```python
from build123d import *

# Parameters (mm, degrees)
SKETCH_R          = 2
PAD_DEPTH         = 8
SKETCH001_R       = 3.05
POCKET_DEPTH      = 0.001
POCKET_DEPTH_BACK = 8.001


with BuildPart() as part:
    # Sketch → Pad (new body)
    with BuildSketch(Plane.XY):
        with BuildLine():
            Line((-54.9, 9), (24.9, 9))
            ThreePointArc((26.9, 7), (26.314214, 8.414214), (24.9, 9))
            Line((26.9, 7), (26.9, -14.5))
            ThreePointArc((24.9, -16.5), (26.314214, -15.914214), (26.9, -14.5))
            Line((-54.9, -16.5), (24.9, -16.5))
            ThreePointArc((-56.9, -14.5), (-56.314214, -15.914214), (-54.9, -16.5))
            Line((-56.9, 7), (-56.9, -14.5))
            ThreePointArc((-54.9, 9), (-56.314214, 8.414214), (-56.9, 7))
        make_face()
        with Locations((-11.1, 5.15)):
            Circle(SKETCH_R, mode=Mode.SUBTRACT)
        with Locations((11.1, -5.15)):
            Circle(SKETCH_R, mode=Mode.SUBTRACT)
        with Locations((-50.9, -12.5)):
            Circle(SKETCH_R, mode=Mode.SUBTRACT)
        with Locations((20.9, -12.5)):
            Circle(SKETCH_R, mode=Mode.SUBTRACT)
        with BuildLine():
            ThreePointArc((-53.9, -3), (-50.9, -6), (-47.9, -3))
            Line((-47.9, -3), (-47.9, 3))
            ThreePointArc((-47.9, 3), (-50.9, 6), (-53.9, 3))
            Line((-53.9, -3), (-53.9, 3))
        make_face(mode=Mode.SUBTRACT)
        with BuildLine():
            ThreePointArc((17.9, -3), (20.9, -6), (23.9, -3))
            Line((23.9, -3), (23.9, 3))
            ThreePointArc((23.9, 3), (20.9, 6), (17.9, 3))
            Line((17.9, -3), (17.9, 3))
        make_face(mode=Mode.SUBTRACT)
    extrude(amount=PAD_DEPTH)

    # Sketch001 → Pocket (cut, two sides)
    with BuildSketch(Plane.XY) as pocket_sk:
        with Locations((-50.9, 0)):
            Circle(SKETCH001_R)
        with Locations((20.9, 0)):
            Circle(SKETCH001_R)
    extrude(amount=-POCKET_DEPTH, mode=Mode.SUBTRACT)
    extrude(pocket_sk.sketch, amount=POCKET_DEPTH_BACK, mode=Mode.SUBTRACT)


solid = part.part
```
The listing builds one solid part. Answer for the finished solid, in the listing's coordinates (mm). A direction names the side the tool comes from. Coordinates: 2 decimals unless noted, no trailing zeros. Order: outer loops, then holes, each group sorted by start corner. A loop starts at its lowest first (then second) coordinate and runs counter-clockwise, first axis right, second up. Notation, with made-up numbers: M 76,-30 L 102,-30 A23 cw 102,-19 Z; hole C 22.25,-7 d4. An arc over 180 degrees is marked long. Answer as a JSON object with one key per item and string values. Group by question number.
1. Section D-D on z = 2.25 is taken. Write down the section's boundary in (x, y).
2. Determine the mould class of faces 1 (the flat face through (23.9, 2, 4)), 2 (the cylindrical face through (26.33, 8.4, 3.94)), 3 (the flat face through (17.9, 2, 4)), 4 (the flat face through (-14, -4, 0)) for opening direction X: released by +X, released by -X, zero draft, split by the parting line, or undercut.
3. A tool of negligible diameter and unlimited length cuts with its end or side. For faces 5 (the flat face through (23.9, -2, 4)), 6 (the flat face through (-16, 9, 4)), from which of +Z, -Z, +X, -X, +Y, -Y can it reach the whole face along a straight path? Write none if from no direction.
4. Straight lines are drawn through the part: line 1 (X direction, y = 1.5, z = 1); line 2 (Y direction, x = -50.9, z = 3); line 3 (Y direction, x = 11, z = 3.25). For each, find the intervals that lie inside material, in ascending order.
5. Section A-A on y = -12.5 is taken. Write down the section's boundary in (x, z).
6. Section C-C on x = 11.1 is taken. Write down the section's boundary in (y, z), then the cut area to 3 significant figures.
7. Section B-B on x = -50.9 is taken. Write down the section's boundary in (y, z), then the cut area to 3 significant figures.
8. A flat-ended cylindrical pin translates along its axis: P1, Ø3.5, axis at x = -11.1, y = 5.15, coming from the -Z side. Find the tip coordinate at first contact, or state that the pin passes through.
Values follow:
{
 "1": {"outline": "M -56.9,-14.5 A2 ccw -54.9,-16.5 L 24.9,-16.5 A2 ccw 26.9,-14.5 L 26.9,7 A2 ccw 24.9,9 L -54.9,9 A2 ccw -56.9,7 Z; hole M -53.9,-3 A3 ccw -47.9,-3 L -47.9,-0.55 A3.05 ccw -47.9,0.55 L -47.9,3 A3 ccw -53.9,3 L -53.9,0.55 A3.05 ccw -53.9,-0.55 Z; hole C -50.9,-12.5 d4; hole C -11.1,5.15 d4; hole C 11.1,-5.15 d4; hole M 17.9,-3 A3 ccw 23.9,-3 L 23.9,-0.55 A3.05 ccw 23.9,0.55 L 23.9,3 A3 ccw 17.9,3 L 17.9,0.55 A3.05 ccw 17.9,-0.55 Z; hole C 20.9,-12.5 d4"},
 "2": {"face 1": "undercut", "face 2": "released by +X", "face 3": "undercut", "face 4": "zero draft"},
 "3": {"face 5": "+Z, -Z", "face 6": "+Z, -Z, +X, -X, +Y"},
 "4": {"line 1": "-56.9 to -53.9, -47.9 to 17.9, 23.9 to 26.9", "line 2": "-16.5 to -14.5, -10.5 to -6, 6 to 9", "line 3": "-16.5 to -7.15, -3.15 to 9"},
 "5": {"outline": "M -56.9,0 L -52.9,0 L -52.9,8 L -56.9,8 Z; M -48.9,0 L 18.9,0 L 18.9,8 L -48.9,8 Z; M 22.9,0 L 26.9,0 L 26.9,8 L 22.9,8 Z"},
 "6": {"outline": "M -16.5,0 L -7.15,0 L -7.15,8 L -16.5,8 Z; M -3.15,0 L 9,0 L 9,8 L -3.15,8 Z", "area": "172 mm2"},
 "7": {"outline": "M -16.5,0 L -14.5,0 L -14.5,8 L -16.5,8 Z; M -10.5,0 L -6,0 L -6,8 L -10.5,8 Z; M 6,0 L 9,0 L 9,8 L 6,8 Z", "area": "76.0 mm2"},
 "8": {"P1": "through"}
}
